```python
from build123d import *

# Parameters (mm, degrees)
SKETCH1_W             = 10
SKETCH1_H             = 5
BOSS_EXTRUDE1_DEPTH   = 21
BOSS_EXTRUDE1_2_DEPTH = 21
SKETCH2_W             = 61
SKETCH2_H             = 43
BOSS_EXTRUDE2_DEPTH   = 5
SKETCH3_W             = 20.5
SKETCH3_H             = 5
BOSS_EXTRUDE3_DEPTH   = 21
CUT_EXTRUDE1_REACH    = 74.498
SKETCH4_R             = 2.2
CUT_EXTRUDE2_REACH    = 77.24
SKETCH5_R             = 1.75
CUT_EXTRUDE4_START    = -5
CUT_EXTRUDE4_DEPTH    = 5
SKETCH11_W            = 5
SKETCH11_H            = 32
BOSS_EXTRUDE5_DEPTH   = 20
SKETCH14_W            = 10
SKETCH14_H            = 5
BOSS_EXTRUDE6_DEPTH   = 6


# Read off the part's stored shape, not the designer's step: Cut-Extrude4
with BuildPart() as part:
    # Sketch1 → Boss-Extrude1 (new body)
    with BuildSketch(Plane(origin=(0, 0, 0), x_dir=(1, 0, 0), z_dir=(0, 1, 0))):
        Rectangle(SKETCH1_W, SKETCH1_H)
    extrude(amount=BOSS_EXTRUDE1_DEPTH)



with BuildPart() as body_2:
    # Sketch1 → Boss-Extrude1 2 (new body)
    with BuildSketch(Plane(origin=(0, 0, 0), x_dir=(1, 0, 0), z_dir=(0, 1, 0))):
        with Locations((51, 0)):
            Rectangle(SKETCH1_W, SKETCH1_H)
    extrude(amount=BOSS_EXTRUDE1_2_DEPTH)


with BuildPart() as part_1:
    add(part.part)

    add(body_2.part)  # Boss-Extrude2 merges body 2
    # Sketch2 → Boss-Extrude2 (add)
    with BuildSketch(Plane(origin=(0, 21, 0), x_dir=(1, 0, 0), z_dir=(0, 1, 0))):
        with Locations((25.5, 19)):
            Rectangle(SKETCH2_W, SKETCH2_H)
    extrude(amount=BOSS_EXTRUDE2_DEPTH)

    # Sketch3 → Boss-Extrude3 (add)
    with BuildSketch(Plane.XZ.offset(-21)):
        with Locations((35.75, -38)):
            Rectangle(SKETCH3_W, SKETCH3_H)
    extrude(amount=BOSS_EXTRUDE3_DEPTH)

    # Sketch4 → Cut-Extrude1 (cut, up to next)
    with BuildSketch(Plane.XY.offset(-35.5), mode=Mode.PRIVATE) as cut_extrude1_sk1:
        with Locations((35.75, 10.5)):
            Circle(SKETCH4_R)
    cut_extrude1_tool1 = extrude(cut_extrude1_sk1.sketch, amount=-CUT_EXTRUDE1_REACH, mode=Mode.PRIVATE) & part_1.part
    add(cut_extrude1_tool1.solids().sort_by_distance((35.75, 10.5, -35.5))[0], mode=Mode.SUBTRACT)

    # Sketch5 → Cut-Extrude2 (cut, up to next)
    with BuildSketch(Plane.XY.offset(2.5), mode=Mode.PRIVATE) as cut_extrude2_sk1:
        with Locations((1.5, 15.5)):
            Circle(SKETCH5_R)
    cut_extrude2_tool1 = extrude(cut_extrude2_sk1.sketch, amount=-CUT_EXTRUDE2_REACH, mode=Mode.PRIVATE) & part_1.part
    # Sketch5 → Cut-Extrude2 (cut, up to next)
    with BuildSketch(Plane.XY.offset(2.5), mode=Mode.PRIVATE) as cut_extrude2_sk2:
        with Locations((49.5, 15.5)):
            Circle(SKETCH5_R)
    cut_extrude2_tool2 = extrude(cut_extrude2_sk2.sketch, amount=-CUT_EXTRUDE2_REACH, mode=Mode.PRIVATE) & part_1.part
    # Sketch5 → Cut-Extrude2 (cut, up to next)
    with BuildSketch(Plane.XY.offset(2.5), mode=Mode.PRIVATE) as cut_extrude2_sk3:
        with Locations((49.5, 5.5)):
            Circle(SKETCH5_R)
    cut_extrude2_tool3 = extrude(cut_extrude2_sk3.sketch, amount=-CUT_EXTRUDE2_REACH, mode=Mode.PRIVATE) & part_1.part
    # Sketch5 → Cut-Extrude2 (cut, up to next)
    with BuildSketch(Plane.XY.offset(2.5), mode=Mode.PRIVATE) as cut_extrude2_sk4:
        with Locations((1.5, 5.5)):
            Circle(SKETCH5_R)
    cut_extrude2_tool4 = extrude(cut_extrude2_sk4.sketch, amount=-CUT_EXTRUDE2_REACH, mode=Mode.PRIVATE) & part_1.part
    add(cut_extrude2_tool1.solids().sort_by_distance((1.5, 15.5, 2.5))[0], mode=Mode.SUBTRACT)
    add(cut_extrude2_tool2.solids().sort_by_distance((49.5, 15.5, 2.5))[0], mode=Mode.SUBTRACT)
    add(cut_extrude2_tool3.solids().sort_by_distance((49.5, 5.5, 2.5))[0], mode=Mode.SUBTRACT)
    add(cut_extrude2_tool4.solids().sort_by_distance((1.5, 5.5, 2.5))[0], mode=Mode.SUBTRACT)

    # Cut-Extrude4 outline → Cut-Extrude4 (cut)
    with BuildSketch(Plane.XZ.offset(-21).offset(CUT_EXTRUDE4_START)):
        with BuildLine():
            Line((25.5, -40.5), (25.5, -35.5))
            add(Edge.make_bspline(
                [(25.5, -35.5), (22.307194013, -9.111827573), (-5, -8.5)],
                knots=[0, 0, 0, 1, 1, 1], degree=2))
            Line((-5, -8.5), (-5, -40.5))
            Line((-5, -40.5), (25.5, -40.5))
        make_face()
        with BuildLine():
            Line((46, -35.5), (46, -40.5))
            Line((46, -40.5), (56, -40.5))
            Line((56, -40.5), (56, -8.5))
            add(Edge.make_bspline(
                [(46, -35.5), (46.761539252, -20.151458346), (56, -8.5)],
                knots=[0, 0, 0, 1, 1, 1], degree=2))
        make_face()
        with BuildLine():
            add(Edge.make_bspline(
                [(31.343896349, -27.5), (31.33756892, -27.477004827), (30.705752309, -25.187905516), (29.116883998, -20.825539694), (25.674792213, -15.02454609), (21.148134772, -10.119526716), (17.495807629, -7.576251466), (15.551950813, -6.5)],
                knots=[0.123732118, 0.123732118, 0.123732118, 0.123732118, 0.125, 0.25, 0.375, 0.5, 0.624358146, 0.624358146, 0.624358146, 0.624358146], degree=3))
            Line((31.343896349, -27.5), (39.715207905, -27.5))
            add(Edge.make_bspline(
                [(39.715207905, -27.5), (39.769177374, -27.217759906), (40.375135311, -24.177689148), (42.00944543, -18.53264277), (44.988088874, -12.248553286), (47.445071003, -8.34732733), (48.500497039, -6.84736316), (48.751036225, -6.5)],
                knots=[0.224487405, 0.224487405, 0.224487405, 0.224487405, 0.25, 0.5, 0.75, 0.875, 0.913034357, 0.913034357, 0.913034357, 0.913034357], degree=3))
            Line((48.751036225, -6.5), (15.551950813, -6.5))
        make_face()
    extrude(amount=CUT_EXTRUDE4_DEPTH, mode=Mode.SUBTRACT)

    # Sketch11 → Boss-Extrude5 (add)
    with BuildSketch(Plane.ZY.offset(5)):
        with Locations((0, 10)):
            Rectangle(SKETCH11_W, SKETCH11_H)
    extrude(amount=BOSS_EXTRUDE5_DEPTH)

    # Sketch14 → Boss-Extrude6 (add)
    with BuildSketch(Plane.XZ):
        Rectangle(SKETCH14_W, SKETCH14_H)
    extrude(amount=BOSS_EXTRUDE6_DEPTH)


solid = part_1.part
```
Source: CAD feature listing. Evaluate the final solid. Frame: model axes, mm. A direction names the side the tool comes from. Coordinates: 2 decimals unless noted, no trailing zeros. Loops run counter-clockwise (first coordinate to the right, second up) from the corner with the lowest first, then second, coordinate; pieces in that order, holes last. Notation, with made-up numbers: M 59.25,15 L 97.25,15 A35 ccw 97.25,50 Z; hole C -5,2.25 d11. An arc over 180 degrees is marked long. Use CSV: the item, a comma, the result in double quotes.
(1) Reachability of faces 1 (the face through (25.5, 13, -38)), 2 (the face through (33, 11, -35.5)), 3 (the face through (46, 13, -38)) from +Z, -Z, +X, -X, +Y, -Y: full face, straight path, thin tool, end or side. Return the list, or none.
Answers follow:
face 1,"-Z, -X, +Y, -Y"
face 2,"+Z, +X, -X, -Y"
face 3,"-Z, +X, +Y, -Y"
(2) Cut plane D-D on y = 20. Return loops of the section in (x, z), and give its area (4 significant figures).
Answers follow:
outline,"M -25,-2.5 L 5,-2.5 L 5,2.5 L -25,2.5 Z; M 25.5,-40.5 L 46,-40.5 L 46,-35.5 L 25.5,-35.5 Z; M 46,-2.5 L 56,-2.5 L 56,2.5 L 46,2.5 Z"
area,"302.5 mm²"
(3) Cut plane B-B on y = 5.5. Return loops of the section in (x, z).
Answers follow:
outline,"M -25,-2.5 L -0.25,-2.5 L -0.25,2.5 L -25,2.5 Z; M 3.25,-2.5 L 5,-2.5 L 5,2.5 L 3.25,2.5 Z; M 25.5,-40.5 L 46,-40.5 L 46,-35.5 L 25.5,-35.5 Z; M 46,-2.5 L 47.75,-2.5 L 47.75,2.5 L 46,2.5 Z; M 51.25,-2.5 L 56,-2.5 L 56,2.5 L 51.25,2.5 Z"
(4) Contact query for flat-ended pins moving along their axis: pin 1 (2 mm diameter, centred on x = 49.5, y = 5.5, fed in from -Z); pin 2 (4 mm diameter, centred on x = 50.5, z = -1, fed in from -Y); pin 3 (1.5 mm diameter, centred on y = 16.5, z = -37.5, fed in from +X); pin 4 (5.5 mm diameter, centred on y = 17, z = -37.5, fed in from -X). Output: stop coordinate, or through.
Answers follow:
pin 1,"through"
pin 2,"y = 0"
pin 3,"x = 46"
pin 4,"x = 25.5"
(5) Line query: line 1 (X direction, y = 13, z = -0.5); line 2 (Y direction, x = 1.5, z = 0.55); line 3 (Y direction, x = 0, z = -1). Output: solid intervals per line, ascending. Write a range as [from, to].
Answers follow:
line 1,"[-25, 5], [46, 56]"
line 2,"[-6, 3.75], [7.25, 13.75], [17.25, 26]"
line 3,"[-6, 4.6], [6.4, 14.6], [16.4, 26]"
(6) Draft query along Y for faces 4 (the face through (25, 21, -17)), 5 (the face through (51, 10, -2.5)), 6 (the face through (1.272, 17.235, 0.035)). Return one class per face: pulls with the +Y half, pulls with the -Y half, needs draft (parallel to the pull), parting line crosses it, or undercut.
Answers follow:
face 4,"pulls with the -Y half"
face 5,"needs draft"
face 6,"undercut"
(7) Cut plane C-C on x = 35.75. Return loops of the section in (y, z).
Answers follow:
outline,"M 0,-40.5 L 8.3,-40.5 L 8.3,-35.5 L 0,-35.5 Z; M 12.7,-40.5 L 26,-40.5 L 26,-27.5 L 21,-27.5 L 21,-35.5 L 12.7,-35.5 Z; M 21,-6.5 L 26,-6.5 L 26,2.5 L 21,2.5 Z"
(8) Cut plane A-A on y = 10.5. Return loops of the section in (x, z).
Answers follow:
outline,"M -25,-2.5 L 5,-2.5 L 5,2.5 L -25,2.5 Z; M 25.5,-40.5 L 33.55,-40.5 L 33.55,-35.5 L 25.5,-35.5 Z; M 37.95,-40.5 L 46,-40.5 L 46,-35.5 L 37.95,-35.5 Z; M 46,-2.5 L 56,-2.5 L 56,2.5 L 46,2.5 Z"
